The model under review builds one solid part; all positions refer to its coordinate system, in mm. A direction names the side the tool comes from. Round coordinates to 2 decimals unless told otherwise and drop trailing zeros. Write each loop counter-clockwise with the first axis right and the second up, starting at its lowest first coordinate (ties: lowest second). Pieces come first, ordered by that corner, then holes. Notation, with made-up numbers: (23.25, -27) -> (36.25, -27) arc R19 ccw to (36.25, -17) -> close; hole circle Ø10 at (-2.75, 67.5). An arc over 180 degrees is marked (long way). Use CSV: the item, a comma, the result in double quotes. Start each with the question number.
1) Take a section at B-B, the plane x = -11. Give the boundary of the cut face in (y, z), then the cut area to 3 significant figures.
2) Mouldability with a two-part tool opening along Y and no side actions: class faces 3 (the face through (-18, 0, 2)), 4 (the face through (0, -2, 0)), 5 (the face through (-1.726, -0.76, -1.293)) as released by +Y, released by -Y, zero draft, split by the parting line, or undercut.
3) Take a section at C-C, the plane x = -18. Give the boundary of the cut face in (y, z), then the cut area to 3 significant figures.
4) Take a section at A-A, the plane z = 0. Give the boundary of the cut face in (x, y).
5) Wall thickness on probe 1 along Y at (x, z) = (-12.5, -2.45); probe 2 along X at (y, z) = (-0.95, 0.2); probe 3 along Y at (x, z) = (-1.5, -0.65): over which ranges is each line inside the solid? List them lowest first. Write a range as [from, to].
6) Machinability: for faces 1 (the face through (-8, -3, 0)), 2 (the face through (-1.726, -0.74, 1.305)), which of the approach directions +Z, -Z, +X, -X, +Y, -Y give a long, thin tool a straight path to every point of the face, cutting with its end or side? Answer none if there is none.
7) For pin 1 Ø1.9 at (x, z) = (-1.5, 0.5) entering from +Y; pin 2 Ø2 at (x, y) = (-13, -2) entering from -Z; pin 3 Ø2 at (x, y) = (-10, 2) entering from +Z, all flat-tipped, find the tip position at first contact; note any pin that passes through.
from build123d import *

# Parameters (mm, degrees)
CUT_EXTRUDE1_DEPTH = 3.5
CHAMFER1_SIZE      = 0.5
CHAMFER1_SIZE2     = 0.288675135


with BuildPart() as part:
    # Sketch1 → Revolve1 (revolve)
    with BuildSketch(Plane.XY):
        Polygon((0, 0), (0, 3), (-15.75, 3), (-16.75, 2), (-20, 2), (-20, 0), align=None)
    revolve(axis=Axis((0, 0, 0), (-1, 0, 0)))

    # Sketch2 → Cut-Extrude1 (cut)
    with BuildSketch(Plane(origin=(0, 0, 0), x_dir=(0, 0, -1), z_dir=(1, 0, 0))):
        Polygon((1.732050808, 0), (0.866025404, 1.5), (-0.866025404, 1.5), (-1.732050808, 0), (-0.866025404, -1.5), (0.866025404, -1.5), align=None)
    extrude(amount=-CUT_EXTRUDE1_DEPTH, mode=Mode.SUBTRACT)

    # Chamfer1
    chamfer1_edges = [part.edges().sort_by_distance(p)[0] for p in [
        (0, -3, 0),
    ]]
    chamfer1_side = [part.faces().sort_by_distance(p)[0] for p in [
        (0, -2.915147186, 0),
    ]]
    chamfer(chamfer1_edges, length=CHAMFER1_SIZE, length2=CHAMFER1_SIZE2, reference=chamfer1_side[0])


solid = part.part
Values found:
1,outline,"circle Ø6 at (0, 0)"
1,area,"28.3 mm²"
2,face 3,"split by the parting line"
2,face 4,"zero draft"
2,face 5,"undercut"
3,outline,"circle Ø4 at (0, 0)"
3,area,"12.6 mm²"
4,outline,"(-20, -2) -> (-16.75, -2) -> (-15.75, -3) -> (-0.29, -3) -> (0, -2.5) -> (0, -1.5) -> (-3.5, -1.5) -> (-3.5, 1.5) -> (0, 1.5) -> (0, 2.5) -> (-0.29, 3) -> (-15.75, 3) -> (-16.75, 2) -> (-20, 2) -> close"
5,probe 1,"[-1.73, 1.73]"
5,probe 2,"[-20, -3.5]"
5,probe 3,"[-2.93, -1.5], [1.5, 2.93]"
6,face 1,"+X, -X"
6,face 2,"+X"
7,pin 1,"y = 3"
7,pin 2,"z = -2.83"
7,pin 3,"z = 2.83"
